Could you check a few things on this drawing? It's one solid part, dimensions in mm from its lowest x, y, z. Give positions to 0.01 mm unless a question says otherwise; leave off trailing zeros. Write each loop counter-clockwise with the first axis right and the second up, starting at its lowest first coordinate (ties: lowest second). Pieces come first, ordered by that corner, then holes. Notation, with made-up numbers: M -0.75,78 L 42.25,78 A22 cw 42.25,96 Z; hole C -32.75,69 d1. An arc over 180 degrees is marked long. Write each question's results on one line, items separated by ' | '.
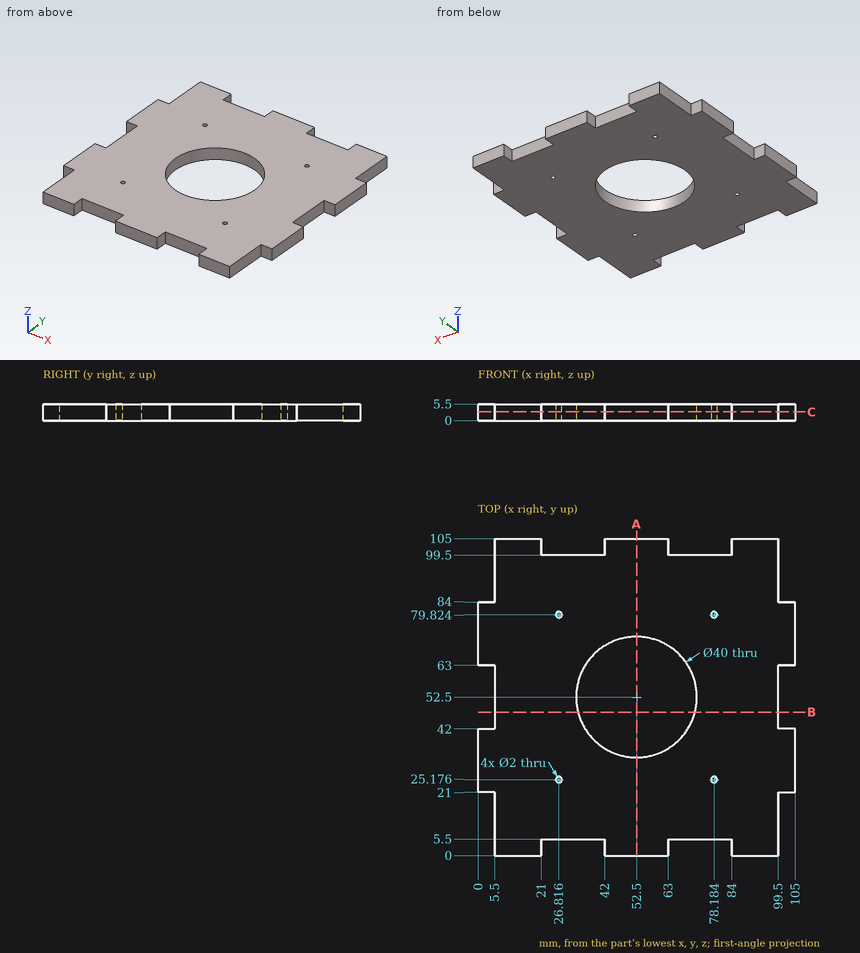
Item 1: I want a section at C-C, the plane z = 2.9. Give the number of separate pieces and of enclosed holes in the cut face, and give its area (3 significant figures).
Geometry says:
separate pieces: 1 | enclosed holes: 5 | area: 8,600 mm2
Item 2: I want a section at A-A, the plane x = 52.5. Please give me the cut outline in (y, z).
Geometry says:
outline: M 0,0 L 32.5,0 L 32.5,5.5 L 0,5.5 Z; M 72.5,0 L 105,0 L 105,5.5 L 72.5,5.5 Z
Item 3: If I drill on line 1 (Y direction, x = 100, z = 1.8); line 2 (Y direction, x = 52.5, z = 1.65); line 3 (Y direction, x = 26.5, z = 2.45) (1 decimal), over which ranges is the centre line in solid material (lowest first)? Write a range as from..to.
Geometry says:
line 1: y = 21..42, 63..84 | line 2: y = 0..32.5, 72.5..105 | line 3: y = 5.5..24.2, 26.1..78.9, 80.8..99.5
Item 4: I'm going to push flat-ended pins straight in: pin 1 (1.6 mm diameter, centred on y = 55, z = 1.5, fed in from -X); pin 2 (1.6 mm diameter, centred on y = 54.5, z = 3.5, fed in from +X); pin 3 (3 mm diameter, centred on x = 81.5, z = 1, fed in from +Y). Where does each tip first touch, or does it pass through?
Geometry says:
pin 1: stops at x = 5.5 | pin 2: stops at x = 99.5 | pin 3: stops at y = 99.5
Item 5: I want a section at B-B, the plane y = 47.5. Please give me the cut outline in (x, z) (1 decimal).
Geometry says:
outline: M 5.5,0 L 33.1,0 L 33.1,5.5 L 5.5,5.5 Z; M 71.9,0 L 99.5,0 L 99.5,5.5 L 71.9,5.5 Z
